from build123d import *

# Parameters (mm, degrees)
F0_R     = 6
F0_R_2   = 5.0929581789
F1_DEPTH = 5
F2_DEPTH = 10
F3_R     = 6
F3_R_2   = 5.0929581789
F4_DEPTH = 0.5
F5_D     = 4.4


with BuildPart() as f1:
    # F0 (on Top) → F1 (new body)
    with BuildSketch(Plane.XY):
        Circle(F0_R)
        Circle(F0_R_2, mode=Mode.SUBTRACT)
        Circle(F0_R_2)
    extrude(amount=F1_DEPTH)

    # F0 (on Top) → F2 (join)
    with BuildSketch(Plane.XY):
        Circle(F0_R_2)
    extrude(amount=F2_DEPTH)

    # F3 (on face) → F4 (join)
    with BuildSketch(Plane.XY.offset(10)):
        Circle(F3_R)
        Circle(F3_R_2, mode=Mode.SUBTRACT)
        Circle(F3_R_2)
    extrude(amount=-F4_DEPTH)

    # F5 (through all)
    with Locations(Plane(origin=(0, 0, 0), x_dir=(1, 0, 0), z_dir=(0, 0, -1))):
        with Locations((0, 0)):
            Hole(F5_D / 2)


solid = f1.part
For this review, take the finished solid that the model builds, in its own axes (mm). A direction names the side the tool comes from. Coordinates: 2 decimals unless noted, no trailing zeros. Order: outer loops, then holes, each group sorted by start corner. A loop starts at its lowest first (then second) coordinate and runs counter-clockwise, first axis right, second up. Notation, with made-up numbers: (-36.75, 35) - (-12.75, 35) arc R30 cw to (-12.75, 74) - close; hole circle Ø5 at (10, 18.25). An arc over 180 degrees is marked (long way). Use one line per item in the form item = value.
Q1. Consider section C-C (z = 6.5). Give the boundary of the cut face in (x, y).
Checked values:
outline = circle Ø10.19 at (0, 0); hole circle Ø4.4 at (0, 0)
Q2. For P1, Ø5, axis at x = -4, z = 1, coming from the +Y side, flat-tipped, find the tip position at first contact; note if it passes through.
Checked values:
P1 = 5.81
Q3. Consider section D-D (x = 3). Give the boundary of the cut face in (y, z), then the cut area to 3 significant figures.
Checked values:
outline = (-5.2, 0) - (5.2, 0) - (5.2, 5) - (4.12, 5) - (4.12, 9.5) - (5.2, 9.5) - (5.2, 10) - (-5.2, 10) - (-5.2, 9.5) - (-4.12, 9.5) - (-4.12, 5) - (-5.2, 5) - close
area = 94.2 mm2
Q4. Consider section A-A (x = 0). Give the boundary of the cut face in (y, z).
Checked values:
outline = (-6, 0) - (-2.2, 0) - (-2.2, 10) - (-6, 10) - (-6, 9.5) - (-5.09, 9.5) - (-5.09, 5) - (-6, 5) - close; (2.2, 0) - (6, 0) - (6, 5) - (5.09, 5) - (5.09, 9.5) - (6, 9.5) - (6, 10) - (2.2, 10) - close
Q5. For probe 1 along Y at (x, z) = (0, 4); probe 2 along Z at (x, y) = (0, 5.5); probe 3 along Y at (x, z) = (0, 7.25), list the stretches that pass through material, from the lowest coordinate up. Write a range as from..to.
Checked values:
probe_1 = -6..-2.2, 2.2..6
probe_2 = 0..5, 9.5..10
probe_3 = -5.09..-2.2, 2.2..5.09
Q6. For faces 1 (the flat face through (-2, -5, 5)), 2 (the cylindrical face through (-6, 0, 2)), list the 3-axis set-ups (+Z, -Z, +X, -X, +Y, -Y) from which the entire face can be reached by the end or side of a thin tool; tool diameter is ignored.
Checked values:
face_1 = none
face_2 = +Z, -Z
Q7. Draft analysis for pull direction Z (two halves, no side actions). For faces 3 (the flat face through (3, 0, 0)), 4 (the flat face through (-2, -5, 9.5)), 5 (the flat face through (3, 0, 10)), state which applies: +Z half, -Z half, draft (parallel to the pull), parting line (faces both ways), or undercut.
Checked values:
face_3 = -Z half
face_4 = undercut
face_5 = +Z half
